Could you check a few things on this model? Use its own coordinates, in mm. A direction names the side the tool comes from. Give positions to 0.01 mm unless a question says otherwise; leave off trailing zeros. Loops run counter-clockwise (first coordinate to the right, second up) from the corner with the lowest first, then second, coordinate; pieces in that order, holes last.
1. Imagine slicing it at A-A (z = 13.5). Count the separate pieces of the cut face and the enclosed holes in it, plus the area to 3 significant figures.
2. Thinking about a two-plate mould opening in X: for faces 1 (the flat face through (-329, 300, 10)), 2 (the cylindrical face through (-537.763, 90.037, 10.14)), 3 (the cylindrical face through (-539.2, 133.2, 10.1)), 4 (the flat face through (-698.747, 148, 10)), which applies, +X half, -X half, draft (parallel to the pull), parting line (faces both ways), or undercut?
3. For faces 5 (the flat face through (-307.247, 79, 10)), 6 (the flat face through (-318, 0, 10)), 7 (the flat face through (-123, 79, 7)), which set-ups out of +Z, -Z, +X, -X, +Y, -Y let a thin tool reach every point of the face, with its end or its side?
4. I need wall thicknesses on line 1 along X through (y, z) = (45, 10.5); line 2 along X through (y, z) = (35, 4.5); line 3 along X through (y, z) = (285, 7.25). Which ranges of each line are inside material? Lowest first, please.
5. Imagine slicing it at B-B (x = -464). List the corners of the cut face in (y, z) for me, plus the area to 3 significant figures.
Solid Edge part; units mm, degrees
sketch "Sketch1" plane through (0, 0, 0) normal (0, 0, 1) x (1, 0, 0)
  line L0 (-698.7474, 0) -> (-698.7474, 300)
  line L1 (-698.7474, 300) -> (51.2526, 300)
  line L2 (51.2526, 300) -> (51.2526, 0)
  line L3 (51.2526, 0) -> (-698.7474, 0)
extrude "Protrusion1" add sketch "Sketch1" along normal blind 20
sketch "Sketch2" plane through (-48.7474, 100, 20) normal (0, 0, 1) x (1, 0, 0)
  circle A0 centre (-65, 25) radius 45.5
  dimension "D1" = 65
extrude "Cutout1" cut sketch "Sketch2" against normal through all
sketch "Sketch3" plane through (-248.7474, 300, 20) normal (0, 0, 1) x (1, 0, 0)
  circle A0 centre (-240, -169) radius 50.5
  dimension "D1" = 240
extrude "Cutout2" cut sketch "Sketch3" against normal through all
hole "Hole_1" at (-531.1738, 173.4264, 20) direction (0, 0, -1) diameter 13.5 end up to next
hole "Hole1" at (-531.1738, 88.5736, 20) direction (0, 0, -1) diameter 13.5 end up to next
hole "Hole2" at (-446.321, 88.5736, 20) direction (0, 0, -1) diameter 13.5 end up to next
hole "Hole3" at (-446.321, 173.4264, 20) direction (0, 0, -1) diameter 13.5 end up to next
hole "Hole_5" at (-167.7474, 125, 20) direction (0, 0, -1) diameter 9 end up to next
hole "Hole4" at (-59.7474, 125, 20) direction (0, 0, -1) diameter 9 end up to next
hole "Hole5" at (-113.7474, 71, 20) direction (0, 0, -1) diameter 9 end up to next
hole "Hole6" at (-113.7474, 179, 20) direction (0, 0, -1) diameter 9 end up to next
sketch "Sketch4" plane through (-248.7474, 300, 20) normal (0, 0, 1) x (1, 0, 0)
  circle A0 centre (135, -175) radius 62
extrude "ExtrudedCutout_4" cut sketch "Sketch4" against normal blind 13
sketch "Sketch5" plane through (-248.7474, 300, 20) normal (0, 0, 1) x (1, 0, 0)
  line L0 (-58.5, -169) -> (-58.5, -275)
  arc A0 (-58.5, -275) -> (-46.5, -275) centre (-52.5, -275) ccw
  line L1 (-46.5, -275) -> (-46.5, -169)
  arc A1 (-58.5, -169) -> (-46.5, -169) centre (-52.5, -169) cw
extrude "Cutout3" cut sketch "Sketch5" against normal through all
hole "Hole_9" at (6.2526, 15, 20) direction (0, 0, -1) diameter 6.6 end through all
hole "Hole7" at (-653.7474, 15, 20) direction (0, 0, -1) diameter 6.6 end through all
hole "Hole8" at (-683.7474, 15, 20) direction (0, 0, -1) diameter 6.6 end through all
hole "Hole9" at (-683.7474, 45, 20) direction (0, 0, -1) diameter 6.6 end through all
hole "Hole10" at (-653.7474, 45, 20) direction (0, 0, -1) diameter 6.6 end through all
hole "Hole11" at (6.2526, 45, 20) direction (0, 0, -1) diameter 6.6 end through all
hole "Hole12" at (36.2526, 45, 20) direction (0, 0, -1) diameter 6.6 end through all
hole "Hole13" at (36.2526, 255, 20) direction (0, 0, -1) diameter 6.6 end through all
hole "Hole14" at (6.2526, 255, 20) direction (0, 0, -1) diameter 6.6 end through all
hole "Hole15" at (-653.7474, 255, 20) direction (0, 0, -1) diameter 6.6 end through all
hole "Hole16" at (-683.7474, 255, 20) direction (0, 0, -1) diameter 6.6 end through all
hole "Hole17" at (-683.7474, 285, 20) direction (0, 0, -1) diameter 6.6 end through all
hole "Hole18" at (-653.7474, 285, 20) direction (0, 0, -1) diameter 6.6 end through all
hole "Hole19" at (6.2526, 285, 20) direction (0, 0, -1) diameter 6.6 end through all
hole "Hole20" at (36.2526, 285, 20) direction (0, 0, -1) diameter 6.6 end through all
hole "Hole21" at (36.2526, 15, 20) direction (0, 0, -1) diameter 6.6 end through all
hole "Hole_25" at (-488.7474, 280, 0) direction (0, 0, 1) diameter 9 end up to next
hole "Hole22" at (-488.7474, 240, 0) direction (0, 0, 1) diameter 9 end up to next
hole "Hole23" at (-448.7474, 240, 0) direction (0, 0, 1) diameter 9 end up to next
hole "Hole24" at (-448.7474, 280, 0) direction (0, 0, 1) diameter 9 end up to next
properties material "Aluminum, 6061-T6"
Derived:
1. separate pieces: 1
1. enclosed holes: 27
1. area: 202,000 mm2
2. face 1: draft
2. face 2: undercut
2. face 3: undercut
2. face 4: -X half
3. face 5: +Z, -Z
3. face 6: +Z, -Z, +X, -X, -Y
3. face 7: +Z
4. line 1: x = -698.75 to -687.05, -680.45 to -657.05, -650.45 to -307.25, -295.25 to 2.95, 9.55 to 32.95, 39.55 to 51.25
4. line 2: x = -698.75 to -307.25, -295.25 to 51.25
4. line 3: x = -698.75 to -687.05, -680.45 to -657.05, -650.45 to 2.95, 9.55 to 32.95, 39.55 to 51.25
5. outline: (0, 0) - (86.98, 0) - (86.98, 20) - (0, 20) - close; (175.02, 0) - (300, 0) - (300, 20) - (175.02, 20) - close
5. area: 4,240 mm2
